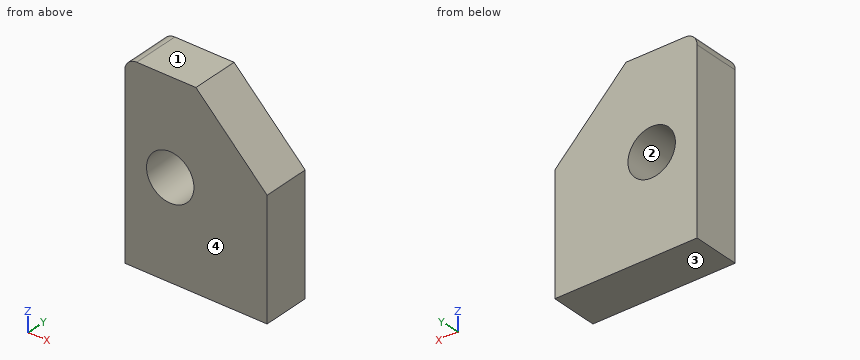
from build123d import *

# Parameters (mm, degrees)
F1_DEPTH = 25.4
F2_SIZE  = 38.1
F3_R     = 12.7
F4_DEPTH = 86.614


with BuildPart() as f1:
    # F0 (on Front) → F1 (new body)
    with BuildSketch(Plane.XZ):
        with BuildLine():
            Line((37.223521, 61.761211), (-32.626479, 61.761211))
            ThreePointArc((-32.626479, 61.761211), (-37.116607, 59.901339), (-38.976479, 55.411211))
            Line((-38.976479, 55.411211), (-38.976479, -39.838789))
            Line((-38.976479, -39.838789), (37.223521, -39.838789))
            Line((37.223521, -39.838789), (37.223521, 61.761211))
        make_face()
    extrude(amount=F1_DEPTH)

    # F2
    f2_edges = [f1.edges().sort_by_distance(p)[0] for p in [
        (37.223521, -12.7, 61.761211),
    ]]
    chamfer(f2_edges, length=F2_SIZE)

    # F3 (on face) → F4 (cut)
    with BuildSketch(Plane.XZ.offset(25.4)):
        with Locations((-14.649719, 12.020282)):
            Circle(F3_R)
    extrude(amount=-F4_DEPTH, mode=Mode.SUBTRACT)


solid = f1.part
Can you work these out from the model? Positions are in its coordinate system, mm. Face numbers are marked on the shaded views. Round coordinates to 2 decimals unless told otherwise and drop trailing zeros. Write each loop counter-clockwise with the first axis right and the second up, starting at its lowest first coordinate (ties: lowest second). Pieces come first, ordered by that corner, then holes. Notation, with made-up numbers: M 58,-25 L 114,-25 A33 cw 114,13 Z; hole C -38,22 d3. An arc over 180 degrees is marked long. Use a Markdown table: item, result.
Item 1: If I drill on line 1 along Z through (x, y) = (-13, -12); line 2 along X through (y, z) = (-2.25, 19.5); line 3 along X through (y, z) = (-19.5, 23), over which ranges is the centre line in solid material (lowest first)? Write a range as [from, to].
Found:
| item | result |
|---|---|
| line 1 | z = [-39.84, -0.57], [24.61, 61.76] |
| line 2 | x = [-38.98, -24.91], [-4.39, 37.22] |
| line 3 | x = [-38.98, -21.03], [-8.27, 37.22] |
Item 2: I want a section at C-C (y = -21). List the corners of the cut face in (x, z) for me, and give its area (3 significant figures).
Found:
| item | result |
|---|---|
| outline | M -38.98,-39.84 L 37.22,-39.84 L 37.22,23.66 L -0.88,61.76 L -32.63,61.76 A6.35 ccw -38.98,55.41 Z; hole C -14.65,12.02 d25.4 |
| area | 6,500 mm2 |
Item 3: I want a section at A-A (x = -10.5). List the corners of the cut face in (y, z) for me, and give its area (3 significant figures).
Found:
| item | result |
|---|---|
| outline | M -25.4,-39.84 L 0,-39.84 L 0,0.02 L -25.4,0.02 Z; M -25.4,24.02 L 0,24.02 L 0,61.76 L -25.4,61.76 Z |
| area | 1,970 mm2 |
Item 4: We'd pull the mould along Z, two halves only. Please class the marked faces 1, 2, 3 and 4: released by +Z, released by -Z, zero draft, split by the parting line, or undercut.
Found:
| item | result |
|---|---|
| face 1 | released by +Z |
| face 2 | undercut |
| face 3 | released by -Z |
| face 4 | zero draft |
Item 5: I want a section at B-B (z = 6.5). List the corners of the cut face in (x, y) for me, and give its area (3 significant figures).
Found:
| item | result |
|---|---|
| outline | M -38.98,-25.4 L -26.09,-25.4 L -26.09,0 L -38.98,0 Z; M -3.21,-25.4 L 37.22,-25.4 L 37.22,0 L -3.21,0 Z |
| area | 1,350 mm2 |
Item 6: For pin 1 Ø20.5 at (x, z) = (-14.65, 12.02) entering from +Y; pin 2 Ø8 at (x, y) = (8.5, -6.5) entering from +Z, each with a flat end and sliding along its axis, tell me the tip position at first contact or that it passes through.
Found:
| item | result |
|---|---|
| pin 1 | passes through |
| pin 2 | stops at z = 56.38 |
Item 7: I want a section at D-D (x = 19). List the corners of the cut face in (y, z) for me, and give its area (3 significant figures).
Found:
| item | result |
|---|---|
| outline | M -25.4,-39.84 L 0,-39.84 L 0,41.88 L -25.4,41.88 Z |
| area | 2,080 mm2 |
